Here's how the part is built. I have some questions about the finished solid (model axes, mm). Face numbers are marked on the shaded views. A direction names the side the tool comes from. Round coordinates to 2 decimals unless told otherwise and drop trailing zeros. Write each loop counter-clockwise with the first axis right and the second up, starting at its lowest first coordinate (ties: lowest second). Pieces come first, ordered by that corner, then holes. Notation, with made-up numbers: (-15, -30.75) -> (-3, -30.75) arc R24 cw to (-3, -17.75) -> close; hole circle Ø3 at (-30.5, 62). An arc over 180 degrees is marked (long way). Answer as CSV lines item,"result".
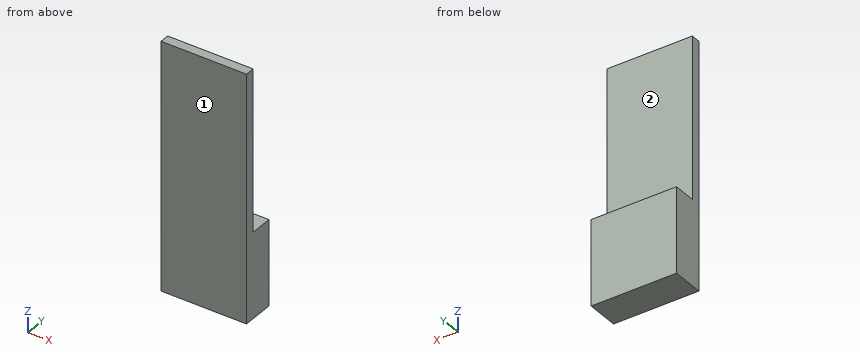
Autodesk Inventor part; units mm, degrees
ref_plane "YZ Plane" through (0, 0, 0) normal (1, 0, 0) x (0, 1, 0)
ref_plane "XZ Plane" through (0, 0, 0) normal (0, 1, 0) x (-1, 0, 0)
ref_plane "XY Plane" through (0, 0, 0) normal (0, 0, 1) x (1, 0, 0)
sketch "Sketch1" plane through (0, 0, 0) normal (0, 1, 0) x (-1, 0, 0)
  line L0 (22.5, 65) -> (-22.5, 65)
  line L1 (-22.5, 65) -> (-22.5, -65)
  line L2 (-22.5, -65) -> (22.5, -65)
  line L3 (22.5, -65) -> (22.5, 65)
  line L4 (22.5, 65) -> (-22.5, -65) construction
  line L5 (-22.5, 65) -> (22.5, -65) construction
  point P0 (0, 0)
  dimension "d0" = 45
  dimension "d1" = 130
extrude "Extrusion1" add sketch "Sketch1" along normal blind 5
sketch "Sketch2" plane through (0, 5, 0) normal (0, 1, 0) x (1, 0, 0)
  line L0 (22.5, 65) -> (-22.5, 65)
  line L1 (22.5, -65) -> (22.5, 65)
  line L2 (-22.5, 65) -> (22.5, 65)
  line L3 (22.5, 65) -> (22.5, 20)
  line L4 (22.5, 20) -> (-22.5, 20)
  line L5 (-22.5, 20) -> (-22.5, 65)
  point P0 (0, 0)
  dimension "d4" = 45
extrude "Extrusion2" add sketch "Sketch2" along normal blind 12
properties part number "linear_motor_base_upper"
Item 1: Suppose I cut it at A-A, the plane x = 17. List the corners of the cut face in (y, z) for me.
Results found:
outline,"(0, -65) -> (17, -65) -> (17, -20) -> (5, -20) -> (5, 65) -> (0, 65) -> close"
Item 2: Suppose I cut it at B-B, the plane y = 10.25. List the corners of the cut face in (x, z) for me.
Results found:
outline,"(-22.5, -65) -> (22.5, -65) -> (22.5, -20) -> (-22.5, -20) -> close"
Item 3: I need wall thicknesses on L1, parallel to Y at x = -8.5, z = 53; L2, parallel to Z at x = -20, y = 6. Which ranges of each line are inside material? Lowest first, please.
Results found:
L1,"y = 0 to 5"
L2,"z = -65 to -20"
Item 4: Will these pins go through, and if not, where does the flat tip stop? pin 1 (5 mm diameter, centred on x = -14, y = 14.5, fed in from +Z); pin 2 (1.5 mm diameter, centred on x = -2.5, z = -2, fed in from +Y); pin 3 (10 mm diameter, centred on y = 14.5, z = 39, fed in from +X).
Results found:
pin 1,"stops at z = -20"
pin 2,"stops at y = 5"
pin 3,"passes through"
Item 5: Suppose I cut it at C-C, the plane z = -15. List the corners of the cut face in (x, y) for me, then the cut area to 3 significant figures.
Results found:
outline,"(-22.5, 0) -> (22.5, 0) -> (22.5, 5) -> (-22.5, 5) -> close"
area,"225 mm²"
Item 6: For the marked faces 1 and 2, which set-ups out of +Z, -Z, +X, -X, +Y, -Y let a thin tool reach every point of the face, with its end or its side?
Results found:
face 1,"+Z, -Z, +X, -X, -Y"
face 2,"+Z, +X, -X, +Y"
